Work out the finished part from the listing and answer in its coordinate system (mm). Face numbers are marked on the shaded views. A direction names the side the tool comes from. Coordinates: 2 decimals unless noted, no trailing zeros. Write each loop counter-clockwise with the first axis right and the second up, starting at its lowest first coordinate (ties: lowest second). Pieces come first, ordered by that corner, then holes. Notation, with made-up numbers: M -38,-4.5 L -10,-4.5 A4 ccw -10,2.5 Z; hole C 43,24 d10. An arc over 180 degrees is marked long. Answer as CSV lines item,"result". Start each with the question number.
(1) For the marked faces 3 and 4, determine the directions among +Z, -Z, +X, -X, +Y, -Y from which every point of the face is accessible in a straight line to the end or side of a thin tool.
(2) A cutting plane is placed at B-B on z = 36.5. Give the vertices of the cut face in (x, y).
(3) Find the intervals of material crossed by L1, parallel to Z at x = -7.5, y = 1; L2, parallel to X at y = -2.5, z = 5; L3, parallel to X at y = -0.5, z = 30.5, in increasing order. Write a range as [from, to].
(4) The mould has two halves that part along Z. Classify the marked faces 1 and 2: released by +Z, released by -Z, zero draft, split by the parting line, or undercut.
(5) A cutting plane is placed at A-A on x = 0. Give the vertices of the cut face in (y, z).
(6) A cutting plane is placed at D-D on x = -3.5. Give the vertices of the cut face in (y, z).
(7) Flat-ended cylindrical pins translate along their axes: P1, Ø6, axis at x = 3.5, z = 5.5, coming from the +Y side; P2, Ø2, axis at y = 6, z = 26, coming from the +X side; P3, Ø10, axis at y = 1.5, z = 37.5, coming from the +X side; P4, Ø2, axis at y = -5.5, z = 27.5, coming from the +X side. Find the tip coordinate at first contact, or state that the pin passes through.
(8) A cutting plane is placed at C-C on y = 4.5. Give the vertices of the cut face in (x, z), then the cut area to 3 significant figures.
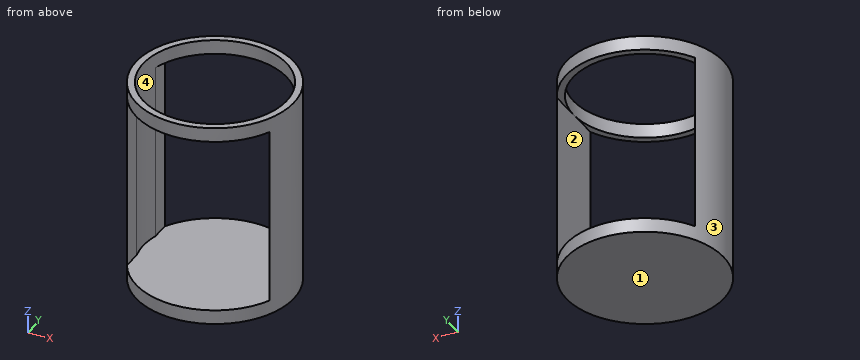
from build123d import *

# Parameters (mm, degrees)
F0_R     = 16.5
F1_DEPTH = 43
F2_R     = 15
F3_DEPTH = 40
F5_W     = 29.508476
F5_H     = 37
F6_DEPTH = 66.501


with BuildPart() as f1:
    # F0 (on Top) → F1 (new body)
    with BuildSketch(Plane.XY):
        Circle(F0_R)
    extrude(amount=F1_DEPTH)

    # F2 (on face) → F3 (cut)
    with BuildSketch(Plane.XY.offset(43)):
        Circle(F2_R)
    extrude(amount=-F3_DEPTH, mode=Mode.SUBTRACT)

    # F5 (on offset) → F6 (cut, through all)
    with BuildSketch(Plane.XZ.offset(50)):
        with Locations((0.245762, 21.5)):
            Rectangle(F5_W, F5_H)
    extrude(amount=-F6_DEPTH, mode=Mode.SUBTRACT)


solid = f1.part
Here are the results:
1,face 3,"+Z, -Z"
1,face 4,"+Z"
2,outline,"M -14.51,-7.86 L -14.51,-3.81 A15 cw -14.51,3.81 L -14.51,7.86 A16.5 ccw Z; M 15,-6.87 A16.5 ccw 15,6.87 Z"
3,L1,"z = [0, 3]"
3,L2,"x = [-16.31, -14.79], [15, 16.31]"
3,L3,"x = [-16.49, -14.99], [15, 16.49]"
4,face 1,"released by -Z"
4,face 2,"undercut"
5,outline,"M -16.5,0 L 16.5,0 L 16.5,3 L -16.5,3 Z; M -16.5,40 L -15,40 L -15,43 L -16.5,43 Z; M 15,40 L 16.5,40 L 16.5,43 L 15,43 Z"
6,outline,"M -16.12,0 L 16.12,0 L 16.12,3 L -16.12,3 Z; M -16.12,40 L -14.59,40 L -14.59,43 L -16.12,43 Z; M 14.59,40 L 16.12,40 L 16.12,43 L 14.59,43 Z"
7,P1,"stops at y = 16.4"
7,P2,"stops at x = 15.72"
7,P3,"stops at x = 16.5"
7,P4,"stops at x = 15.87"
8,outline,"M -15.87,0 L 15.87,0 L 15.87,43 L 14.31,43 L 14.31,40 L 15,40 L 15,3 L -14.51,3 L -14.51,40 L -14.31,40 L -14.31,43 L -15.87,43 Z"
8,area,"188 mm^2"
